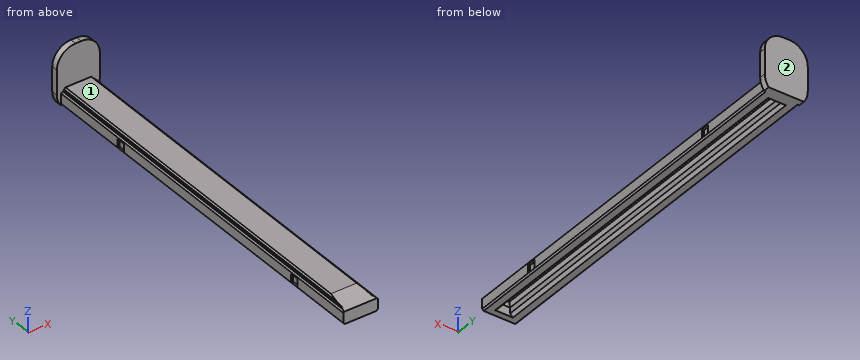
from build123d import *

# Parameters (mm, degrees)
F1_DEPTH = 135
F2_SIZE2 = 8
F2_SIZE  = 1.2
F4_DEPTH = 2.2
F5_W     = 3
F5_H     = 3
F6_DEPTH = 0.7
F7_SIZE  = 0.49999
F8_W     = 4.2
F8_H     = 130.6
F9_DEPTH = 4
F10_SIZE = 1


# Not quite as in the source:
# - a fillet or chamfer is up to 0.001 mm smaller than in the source, because OpenCascade refuses the exact size
# - a pattern or mirror of a feature is missing from the dataset's text; its kind, count and spacing are read off the source's solid


with BuildPart() as f1:
    # F0 (on Front) → F1 (new body)
    with BuildSketch(Plane.XZ):
        Polygon((-6, -2.75), (6, -2.75), (6, 1.75), (5, 1.75), (5, 2.75), (-5, 2.75), (-5, 1.75), (-6, 1.75), align=None)
    extrude(amount=F1_DEPTH)

    # F2
    f2_edges = [f1.edges().sort_by_distance(p)[0] for p in [
        (0, -135, 2.75),
    ]]
    f2_side = f1.faces().sort_by_distance((0, -135, -0.070312))[0]
    chamfer(f2_edges, length=F2_SIZE, length2=F2_SIZE2, reference=f2_side)

    # F3 (on Front) → F4 (join)
    with BuildSketch(Plane.XZ):
        with BuildLine():
            ThreePointArc((7.5, 9.85), (5.5961940777, 14.4461940777), (1, 16.35))
            Line((1, 16.35), (-1, 16.35))
            ThreePointArc((-1, 16.35), (-5.5961940777, 14.4461940777), (-7.5, 9.85))
            Line((-7.5, 9.85), (-7.5, 1.25))
            ThreePointArc((-7.5, 1.25), (-7.1462423475, -0.8651134734), (-6.123475383, -2.75))
            Line((-6.123475383, -2.75), (6.123475383, -2.75))
            ThreePointArc((6.123475383, -2.75), (7.1462423475, -0.8651134734), (7.5, 1.25))
            Line((7.5, 1.25), (7.5, 9.85))
        make_face()
    extrude(amount=-F4_DEPTH)

    # F5 (on face) → F6 (cut)
    with BuildSketch(Plane(origin=(-6, 0, 0), x_dir=(0, -1, 0), z_dir=(-1, 0, 0))):
        with Locations((28.5, -0.75)):
            Rectangle(F5_W, F5_H)
        with Locations((111.5, -0.75)):
            Rectangle(F5_W, F5_H)
    f6 = extrude(amount=-F6_DEPTH, mode=Mode.SUBTRACT)

    # F6_copies: F6 across plane
    add(f6.mirror(Plane(origin=(0, 0, 0), x_dir=(0, 0, 1), z_dir=(1, 0, 0))), mode=Mode.SUBTRACT)

    # F7 (size 0.5 in the source; OpenCascade refuses exactly that, so slightly less here)
    f7_edges = [f1.edges().sort_by_distance(p)[0] for p in [
        (6, -67.5, -2.75),
        (-6, -67.5, -2.75),
        (6, -66.833333, 1.75),
        (5, -63.5, 2.75),
        (-5, -63.5, 2.75),
        (-6, -66.833333, 1.75),
    ]]
    chamfer(f7_edges, length=F7_SIZE)

    # F8 (on face) → F9 (cut)
    with BuildSketch(Plane(origin=(0, 0, -2.75), x_dir=(1, 0, 0), z_dir=(0, 0, -1))):
        with Locations((0, 67.5)):
            Rectangle(F8_W, F8_H)
    extrude(amount=-F9_DEPTH, mode=Mode.SUBTRACT)

    # F10
    f10_edges = [f1.edges().sort_by_distance(p)[0] for p in [
        (0, -132.8, 1.25),
        (-2.1, -67.5, 1.25),
        (2.1, -67.5, 1.25),
        (0, -2.2, 1.25),
        (2.1, -67.5, -2.75),
        (-2.1, -67.5, -2.75),
    ]]
    chamfer(f10_edges, length=F10_SIZE)


solid = f1.part
The model under review builds one solid part; all positions refer to its coordinate system, in mm. Face numbers are marked on the shaded views. A direction names the side the tool comes from. Coordinates: 2 decimals unless noted, no trailing zeros. Loops run counter-clockwise (first coordinate to the right, second up) from the corner with the lowest first, then second, coordinate; pieces in that order, holes last. Notation, with made-up numbers: (-19.75, 2.5) -> (6.25, 2.5) arc R26 cw to (6.25, 39.5) -> close; hole circle Ø5 at (-32.5, -20.5). An arc over 180 degrees is marked (long way). Use a Markdown table: item, result. Add a question column.
1. To check wall thickness, follow line 1 (X direction, y = -86, z = -1.25); line 2 (Y direction, x = -0.5, z = 0); line 3 (Z direction, x = -5.5, y = -8.5). State the ranges of each line that lie inside material, in increasing order.
2. Machinability: for the marked faces 1 and 2, which of the approach directions +Z, -Z, +X, -X, +Y, -Y give a long, thin tool a straight path to every point of the face, cutting with its end or side? Answer none if there is none.
3. Clearance check with flat-ended pins moving along their axes: pin 1 Ø5 at (x, y) = (-2.5, -39.5) entering from +Z; pin 2 Ø4 at (y, z) = (-118.5, 5.5) entering from -X; pin 3 Ø3 at (y, z) = (-68, -0.5) entering from +X; pin 4 Ø0.8 at (x, y) = (-5.5, -112) entering from +Z. State where each tip first meets the part, or that it passes through.
4. Add section A-A on y = -95.5. Write out the cut boundary in (x, z).
5. Add section B-B on z = 4.5. Write out the cut boundary in (x, y), plus the area to 3 significant figures.
Returned:
| question | item | result |
|---|---|---|
| 1 | line 1 | x = -6 to -2.1, 2.1 to 6 |
| 1 | line 2 | y = -135 to -132.8, -2.2 to 2.2 |
| 1 | line 3 | z = -2.75 to 1.75 |
| 2 | face 1 | +Z, +X, -X, -Y |
| 2 | face 2 | +Z, -Z, +X, -X, +Y |
| 3 | pin 1 | stops at z = 2.75 |
| 3 | pin 2 | passes through |
| 3 | pin 3 | stops at x = 6 |
| 3 | pin 4 | stops at z = 1.75 |
| 4 | outline | (-6, -2.25) -> (-5.5, -2.75) -> (-3.1, -2.75) -> (-2.1, -1.75) -> (-2.1, 0.25) -> (-1.1, 1.25) -> (1.1, 1.25) -> (2.1, 0.25) -> (2.1, -1.75) -> (3.1, -2.75) -> (5.5, -2.75) -> (6, -2.25) -> (6, 1.25) -> (5.5, 1.75) -> (5, 1.75) -> (5, 2.25) -> (4.5, 2.75) -> (-4.5, 2.75) -> (-5, 2.25) -> (-5, 1.75) -> (-5.5, 1.75) -> (-6, 1.25) -> close |
| 5 | outline | (-7.5, 0) -> (7.5, 0) -> (7.5, 2.2) -> (-7.5, 2.2) -> close |
| 5 | area | 33.0 mm² |
